Build history of the part. All positions in model axes, mm. A direction names the side the tool comes from. Give positions to 0.01 mm unless a question says otherwise; leave off trailing zeros. Loops run counter-clockwise (first coordinate to the right, second up) from the corner with the lowest first, then second, coordinate; pieces in that order, holes last. Notation, with made-up numbers: (12, 29) -> (28, 29) arc R19 cw to (28, 35) -> close; hole circle Ø6 at (43.25, 18). An arc over 180 degrees is marked (long way). Answer as a JSON object with one key per item and string values. Group by question number.
Q1. Band-saw the part on C-C, the plane y = 80. Write the cut outline in (x, z).
Q2. Band-saw the part on A-A, the plane x = -500. Write the cut outline in (y, z), plus the area to 3 significant figures.
Q3. Band-saw the part on D-D, the plane z = 0. Write the cut outline in (x, y).
Q4. Drop flat-ended pins along their axis: pin 1 (8 mm diameter, centred on y = 24.5, z = 91.5, fed in from -X); pin 2 (3 mm diameter, centred on x = -724, z = 112, fed in from -Y). Give the stop position or say it passes through.
Q5. Tool access for faces 3 (the flat face through (0, 0, 0)), 4 (the cylindrical face through (-822.796, 93.374, 122.97)), 5 (the cylindrical face through (-511.55, 10.33, -7.37)), 6 (the cylindrical face through (-260.446, -13.583, 1.783)): list every direction of +Z, -Z, +X, -X, +Y, -Y with a clear straight run to the whole face (end or side of a thin tool).
Q6. Two-plate mould, pull along Y, no slides. Class faces 1 (the cylindrical face through (-491.7, 50.6, 130.9)), 2 (the flat face through (-1150, 80, 120)): pulls with the +Y half, pulls with the -Y half, needs draft (parallel to the pull), parting line crosses it, or undercut.
Q7. Wall check: probe 1 along X at (y, z) = (19, 53.5); probe 2 along X at (y, z) = (69, 126); probe 3 along Y at (x, z) = (-1036, 115) (3 decimals). Give the ranges that are in metal, low to high. Write a range as from..to.
Q8. Band-saw the part on B-B, the plane z = 120. Write the cut outline in (x, y), plus the area to 3 significant figures.
from build123d import *

# Parameters (mm, degrees)
CROQUIS1_R = 13.7


with BuildPart() as part:
    # Barrer1: sweep along a curve in space
    with BuildLine() as barrer1_path:
        Line((0, 0, 0), (-500, 0, 0))
        Line((-500, 0, 0), (-500, 20, 0))
        Line((-500, 20, 0), (-500, 20, 120))
        Line((-500, 20, 120), (-500, 80, 120))
        Line((-500, 80, 120), (-1150, 80, 120))
    # Croquis1 → Barrer1 (sweep)
    with BuildSketch(Plane(origin=(0, 0, 0), x_dir=(0, 0, -1), z_dir=(1, 0, 0))):
        Circle(CROQUIS1_R)
    sweep(path=barrer1_path.line, transition=Transition.RIGHT)


solid = part.part
Worked answers:
{
 "1": {"outline": "(-1150, 106.3) -> (-500, 106.3) arc R13.7 ccw to (-500, 133.7) -> (-1150, 133.7) -> close"},
 "2": {"outline": "(0, -13.7) -> (33.7, -13.7) -> (33.7, 106.3) -> (80, 106.3) arc R13.7 ccw to (80, 133.7) -> (6.3, 133.7) -> (6.3, 13.7) -> (0, 13.7) arc R13.7 ccw to start", "area": "6,070 mm2"},
 "3": {"outline": "(-513.7, -13.7) -> (0, -13.7) -> (0, 13.7) -> (-486.3, 13.7) -> (-486.3, 20) arc R13.7 ccw to (-513.7, 20) -> close"},
 "4": {"pin 1": "x = -513.69", "pin 2": "y = 67.94"},
 "5": {"face 3": "+Z, -Z, +X, +Y, -Y", "face 4": "-X", "face 5": "none", "face 6": "+X"},
 "6": {"face 1": "undercut", "face 2": "needs draft"},
 "7": {"probe 1": "-513.66..-486.34", "probe 2": "-1150..-487.68", "probe 3": "67.245..92.755"},
 "8": {"outline": "(-1150, 66.3) -> (-513.7, 66.3) -> (-513.7, 20) arc R13.7 ccw to (-486.3, 20) -> (-486.3, 93.7) -> (-1150, 93.7) -> close", "area": "19,700 mm2"}
}
